For this review, take the finished solid that the model builds, in its own axes (mm). Coordinates: 2 decimals unless noted, no trailing zeros. Order: outer loops, then holes, each group sorted by start corner. A loop starts at its lowest first (then second) coordinate and runs counter-clockwise, first axis right, second up. Notation, with made-up numbers: (55.5, -10) - (79.5, -10) arc R37 ccw to (79.5, 27) - close; hole circle Ø7 at (52, 26.25). An arc over 180 degrees is marked (long way). One line per item, written item: value. Start each with the question number.
(1) Consider section A-A on y = 11. Write out the cut boundary in (x, z).
(2) To check wall thickness, follow line 1 along Y through (x, z) = (0, 1.45); line 2 along Y through (x, z) = (-1, 1.5); line 3 along Y through (x, z) = (5.5, 0.7). State the ranges of each line that lie inside material, in increasing order.
(3) Consider section B-B on y = 37. Write out the cut boundary in (x, z).
(4) Consider section C-C on x = 0. Write out the cut boundary in (y, z).
(5) Clearance check with a flat-ended pin moving along its axis: pin 1 (2.5 mm diameter, centred on x = 0, y = 73, fed in from -Z). State where the tip first meets the part, or that it passes through.
(6) Consider section D-D on z = 1.4. Write out the cut boundary in (x, y).
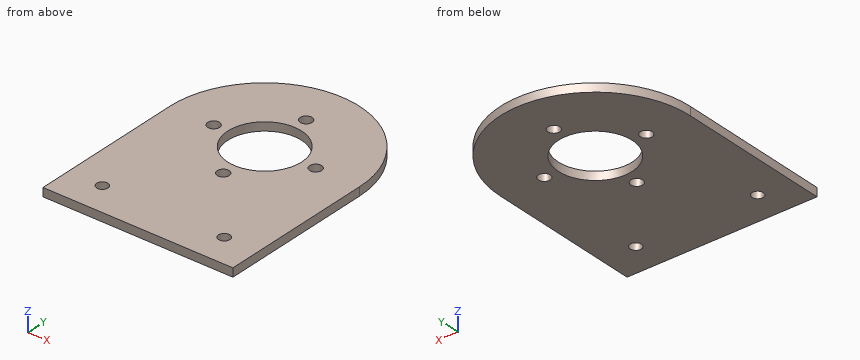
```python
from build123d import *

# Parameters (mm, degrees)
SKETCH1_R           = 13
SKETCH1_R_2         = 2.1
SKETCH1_R_3         = 2
BOSS_EXTRUDE1_DEPTH = 3


with BuildPart() as part:
    # Sketch1 → Boss-Extrude1 (new body)
    with BuildSketch(Plane.XY):
        with BuildLine():
            Line((-33.5, 0), (33.5, 0))
            Line((33.5, 0), (33.5, 55))
            ThreePointArc((33.5, 55), (0, 88.5), (-33.5, 55))
            Line((-33.5, 55), (-33.5, 0))
        make_face()
        with Locations((0, 55)):
            Circle(SKETCH1_R, mode=Mode.SUBTRACT)
        with Locations((0, 37)):
            Circle(SKETCH1_R_2, mode=Mode.SUBTRACT)
        with Locations((-21.5, 11)):
            Circle(SKETCH1_R_3, mode=Mode.SUBTRACT)
        with Locations(Location((21.5, 11, 0), (0, 0, 180))):
            Circle(SKETCH1_R_3, mode=Mode.SUBTRACT)
        with Locations((-18, 55)):
            Circle(SKETCH1_R_2, mode=Mode.SUBTRACT)
        with Locations((0, 73)):
            Circle(SKETCH1_R_2, mode=Mode.SUBTRACT)
        with Locations((18, 55)):
            Circle(SKETCH1_R_2, mode=Mode.SUBTRACT)
    extrude(amount=BOSS_EXTRUDE1_DEPTH)


solid = part.part
```
Geometry check:
1. outline: (-33.5, 0) - (-23.5, 0) - (-23.5, 3) - (-33.5, 3) - close; (-19.5, 0) - (19.5, 0) - (19.5, 3) - (-19.5, 3) - close; (23.5, 0) - (33.5, 0) - (33.5, 3) - (23.5, 3) - close
2. line 1: y = 0 to 34.9, 39.1 to 42, 68 to 70.9, 75.1 to 88.5
2. line 2: y = 0 to 35.15, 38.85 to 42.04, 67.96 to 71.15, 74.85 to 88.49
2. line 3: y = 0 to 43.22, 66.78 to 88.05
3. outline: (-33.5, 0) - (-2.1, 0) - (-2.1, 3) - (-33.5, 3) - close; (2.1, 0) - (33.5, 0) - (33.5, 3) - (2.1, 3) - close
4. outline: (0, 0) - (34.9, 0) - (34.9, 3) - (0, 3) - close; (39.1, 0) - (42, 0) - (42, 3) - (39.1, 3) - close; (68, 0) - (70.9, 0) - (70.9, 3) - (68, 3) - close; (75.1, 0) - (88.5, 0) - (88.5, 3) - (75.1, 3) - close
5. pin 1: passes through
6. outline: (-33.5, 0) - (33.5, 0) - (33.5, 55) arc R33.5 ccw to (-33.5, 55) - close; hole circle Ø4 at (-21.5, 11); hole circle Ø4.2 at (-18, 55); hole circle Ø26 at (0, 55); hole circle Ø4.2 at (0, 37); hole circle Ø4.2 at (0, 73); hole circle Ø4.2 at (18, 55); hole circle Ø4 at (21.5, 11)
